Could you check a few things on this model? Use its own coordinates, in mm. Round coordinates to 2 decimals unless told otherwise and drop trailing zeros. Answer as CSV lines item,"result". Start each with the question number.
1) We'd pull the mould along X, two halves only. Please class faces 1 (the face through (9, 3, 15.8)), 2 (the face through (-1.5, -2, 12)): pulls with the +X half, pulls with the -X half, needs draft (parallel to the pull), parting line crosses it, or undercut.
2) Suppose I cut it at A-A, the plane z = 10. Count the separate pieces of the cut face and the enclosed holes in it, then the cut area to 3 significant figures.
3) I'm going to push flat-ended pins straight in: pin 1 Ø9 at (x, y) = (-1, -8) entering from -Z; pin 2 Ø6 at (y, z) = (-9.5, 10.5) entering from -X; pin 3 Ø12 at (x, y) = (-4, 1) entering from -Z. Where does each tip first touch, or does it pass through?
4) Please list where these lines run through material, in increasing order: line 1 along X through (y, z) = (8, 15.5); line 2 along X through (y, z) = (10.5, 15.75); line 3 along Y through (x, z) = (0, 9.75).
```python
from build123d import *

# Parameters (mm, degrees)
PAD_DEPTH             = 8
SKETCH003_W           = 5.5
SKETCH003_H           = 1
POCKET_DEPTH          = 8
FILLET001_R           = 1
PAD001_DEPTH          = 0.4
POLARPATTERN_COUNT    = 4
POLARPATTERN_ANGLE    = 120
POLARPATTERN001_COUNT = 4
POLARPATTERN001_ANGLE = 120
PAD002_DEPTH          = 0.8


with BuildPart() as part:
    # Sketch → Revolution001 (revolve)
    with BuildSketch(Plane.XZ):
        with BuildLine():
            Line((-15, 17), (0, 17))
            Line((0, 17), (0, 15.8))
            Line((0, 15.8), (-13.4, 15.8))
            add(Edge.make_bspline(
                [(-13.4, 15.8), (-13.6, 4.4), (-15.8, 1.5)],
                knots=[0, 0, 0, 1, 1, 1], degree=2))
            Line((-15.8, 1.5), (-17, 1.5))
            add(Edge.make_bspline(
                [(-15, 17), (-15.191235, 4.567246), (-17, 1.5)],
                knots=[0, 0, 0, 1, 1, 1], degree=2))
        make_face()
    revolve(axis=Axis((0, 0, 0), (0, 0, 1)))

    # Sketch002 (on Face2 of Revolution001) → Pad (new body)
    with BuildSketch(Plane(origin=(0, 0, 15.8), x_dir=(1, 0, 0), z_dir=(0, 0, -1))):
        with BuildLine():
            Line((-2.5, 3.122499), (-2.5, -3.122499))
            ThreePointArc((-2.5, -3.122499), (4, 0), (-2.5, 3.122499))
        make_face()
        with BuildLine():
            Line((-1.5, 2.598076), (-1.5, -2.598076))
            ThreePointArc((-1.5, -2.598076), (3, 0), (-1.5, 2.598076))
        make_face(mode=Mode.SUBTRACT)
    extrude(amount=PAD_DEPTH)

    # Sketch003 (on Face8 of Pad) → Pocket (cut)
    with BuildSketch(Plane(origin=(0, 0, 7.8), x_dir=(1, 0, 0), z_dir=(0, 0, -1))):
        Rectangle(SKETCH003_W, SKETCH003_H)
    extrude(amount=-POCKET_DEPTH, mode=Mode.SUBTRACT)

    # Fillet001
    fillet001_edges = [part.edges().sort_by_distance(p)[0] for p in [
        (15, 0, 17),
    ]]
    fillet(fillet001_edges, radius=FILLET001_R)

    # Sketch004 → Pad001 (join, symmetric)
    with BuildSketch(Plane.XZ):
        Polygon((3.5, 16.2), (14.1, 16.2), (15.3, 4.1), (3.5, 8.1), align=None)
    pad001 = extrude(amount=PAD001_DEPTH, both=True)

    # PolarPattern: Pad001 ×4 about axis
    polarpattern_axis = Axis((0, 0, 0), (0, 0, 1))
    for i in range(1, POLARPATTERN_COUNT):
        add(pad001.rotate(polarpattern_axis, i * POLARPATTERN_ANGLE / (POLARPATTERN_COUNT - 1)))

    # PolarPattern001: Pad001 ×4 about axis
    polarpattern001_axis = Axis((0, 0, 0), (0, 0, -1))
    for i in range(1, POLARPATTERN001_COUNT):
        add(pad001.rotate(polarpattern001_axis, i * POLARPATTERN001_ANGLE / (POLARPATTERN001_COUNT - 1)))

    # Sketch005 (on DatumPlane) → Pad002 (join)
    with BuildSketch(Plane(origin=(0, -1, 0), x_dir=(0.951057, 0.309017, 0), z_dir=(0.309017, -0.951057, 0))):
        Polygon((-2.2, 16.2), (-14.1, 16.2), (-15.3, 4.1), (-2.2, 8.1), align=None)
    pad002 = extrude(amount=-PAD002_DEPTH)

    # Mirrored: Pad002 across XZ
    add(pad002.mirror(Plane.XZ))

    # Sketch006 (on DatumPlane) → Groove (revolve, cut)
    with BuildSketch(Plane.XZ):
        with BuildLine():
            Line((-14.256, 21.131777), (-16.27368, 4.256502))
            add(Edge.make_bspline(
                [(-14.256, 21.131777), (-14.019386, 16.117344), (-14.892639, 6.241907), (-16.27368, 4.256502)],
                knots=[0, 0, 0, 0, 1, 1, 1, 1], degree=3))
        make_face()
    revolve(axis=Axis((-17, 0, 0), (0.121265, 0.000738, 0.99262)), mode=Mode.SUBTRACT)


solid = part.part
```
Filled sheet:
1,face 1,"undercut"
1,face 2,"undercut"
2,separate pieces,"1"
2,enclosed holes,"9"
2,area,"238 mm²"
3,pin 1,"z = 5.3"
3,pin 2,"x = -13.82"
3,pin 3,"z = 5.78"
4,line 1,"-12.72 to -10.76, -5.08 to -4.16, 1 to 1.82, 8.91 to 10.16, 10.76 to 12.72"
4,line 2,"-10.75 to -8.33, -6.52 to -5.6, 1.45 to 2.26, 8.33 to 10.75"
4,line 3,"-15.31 to -13.7, -4 to -3, 3 to 4, 13.7 to 15.31"
